from build123d import *

# Parameters (mm, degrees)
SKETCH1_R           = 1.2
BOSS_EXTRUDE1_DEPTH = 1.5


with BuildPart() as part:
    # Sketch1 → Boss-Extrude1 (new body, symmetric)
    with BuildSketch(Plane.XY):
        with BuildLine():
            Line((-24.40896688, -2.429131501), (-4.150358361, 2.5))
            Line((-4.150358361, 2.5), (4.150358361, 2.5))
            Line((4.150358361, 2.5), (24.40896688, -2.429131501))
            ThreePointArc((24.40896688, -2.429131501), (27.429131501, -0.59103312), (25.59103312, 2.429131501))
            Line((25.59103312, 2.429131501), (5.041156826, 7.429131501))
            ThreePointArc((5.041156826, 7.429131501), (4.747757076, 7.482219647), (4.450123705, 7.5))
            Line((4.450123705, 7.5), (-4.450123705, 7.5))
            ThreePointArc((-4.450123705, 7.5), (-4.747757076, 7.482219647), (-5.041156826, 7.429131501))
            Line((-5.041156826, 7.429131501), (-25.59103312, 2.429131501))
            ThreePointArc((-25.59103312, 2.429131501), (-27.429131501, -0.59103312), (-24.40896688, -2.429131501))
        make_face()
        with Locations((-25, 0)):
            Circle(SKETCH1_R, mode=Mode.SUBTRACT)
        with Locations((25, 0)):
            Circle(SKETCH1_R, mode=Mode.SUBTRACT)
    extrude(amount=BOSS_EXTRUDE1_DEPTH, both=True)


solid = part.part
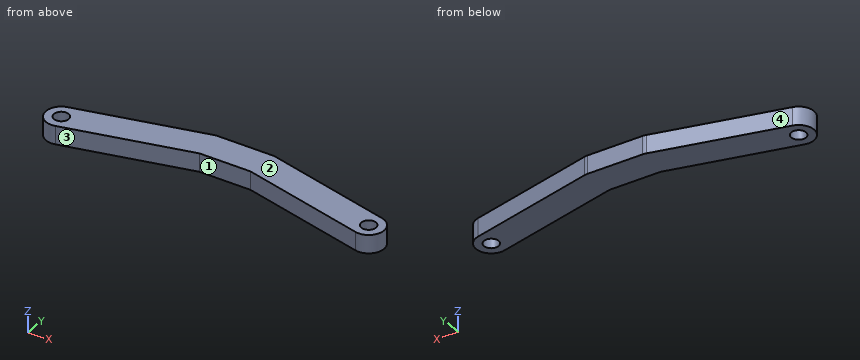
The listing builds one solid part. Answer for the finished solid, in the listing's coordinates (mm). Face numbers are marked on the shaded views. Round coordinates to 2 decimals unless told otherwise and drop trailing zeros. Order: outer loops, then holes, each group sorted by start corner. A loop starts at its lowest first (then second) coordinate and runs counter-clockwise, first axis right, second up. Notation, with made-up numbers: (14.5, -18) -> (19.5, -18) arc R27 ccw to (19.5, 15) -> close; hole circle Ø6 at (21.5, 55.5). An arc over 180 degrees is marked (long way). Put each result on its own line as item: value.
Q1. Consider line 1 along Y through (x, z) = (2, -0.75); line 2 along Y through (x, z) = (-25, 0.7); line 3 along Y through (x, z) = (-19, -0.7). Determine where each line is inside the solid, lowest interval first.
Results list:
line 1: 2.5 to 7.5
line 2: -2.5 to -1.2, 1.2 to 2.57
line 3: -1.11 to 4.03
Q2. Section A-A, the plane z = 0 is taken. Write down the section's boundary in (x, y), and give its area (3 significant figures).
Results list:
outline: (-25.59, 2.43) arc R2.5 ccw to (-24.41, -2.43) -> (-4.15, 2.5) -> (4.15, 2.5) -> (24.41, -2.43) arc R2.5 ccw to (25.59, 2.43) -> (5.04, 7.43) arc R2.5 ccw to (4.45, 7.5) -> (-4.45, 7.5) arc R2.5 ccw to (-5.04, 7.43) -> close; hole circle Ø2.4 at (-25, 0); hole circle Ø2.4 at (25, 0)
area: 267 mm^2
Q3. Section B-B, the plane y = 0 is taken. Write down the section's boundary in (x, z).
Results list:
outline: (-27.5, -1.5) -> (-26.2, -1.5) -> (-26.2, 1.5) -> (-27.5, 1.5) -> close; (-23.8, -1.5) -> (-14.43, -1.5) -> (-14.43, 1.5) -> (-23.8, 1.5) -> close; (14.43, -1.5) -> (23.8, -1.5) -> (23.8, 1.5) -> (14.43, 1.5) -> close; (26.2, -1.5) -> (27.5, -1.5) -> (27.5, 1.5) -> (26.2, 1.5) -> close
Q4. Section C-C, the plane x = 25 is taken. Write down the section's boundary in (y, z), and give its area (3 significant figures).
Results list:
outline: (-2.5, -1.5) -> (-1.2, -1.5) -> (-1.2, 1.5) -> (-2.5, 1.5) -> close; (1.2, -1.5) -> (2.57, -1.5) -> (2.57, 1.5) -> (1.2, 1.5) -> close
area: 8.02 mm^2
Q5. Section D-D, the plane x = 2 is taken. Write down the section's boundary in (y, z), and give its area (3 significant figures).
Results list:
outline: (2.5, -1.5) -> (7.5, -1.5) -> (7.5, 1.5) -> (2.5, 1.5) -> close
area: 15.0 mm^2
Q6. Each of these flat-tipped pins is pushed along its axis until it touches: P1, Ø3, axis at x = -25, y = 0, coming from the +Z side; P2, Ø1.5, axis at x = 6.5, z = -1, coming from the -Y side; P3, Ø1.9, axis at x = 25, y = 0, coming from the -Z side. Where does it stop, or does it pass through?
Results list:
P1: z = 1.5
P2: y = 1.75
P3: through
Q7. Determine the mould class of the marked faces 1, 2, 3 and 4 for opening direction X: pulls with the +X half, pulls with the -X half, needs draft (parallel to the pull), parting line crosses it, or undercut.
Results list:
face 1: undercut
face 2: needs draft
face 3: undercut
face 4: pulls with the -X half
